```python
from build123d import *

# Parameters (mm, degrees)
F0_W          = 177.334
F0_H          = 19.05
F0_R          = 3.1369
F0_R_2        = 4.7625
F1_DEPTH      = 12.7
F2_W          = 177.334
F2_H          = 6.35
F3_DEPTH      = 25.4
F3_DEPTH_BACK = 12.7


with BuildPart() as f1:
    # F0 (on Front) → F1 (new body)
    with BuildSketch(Plane.XZ):
        with Locations((88.667, 9.525)):
            Rectangle(F0_W, F0_H)
        with Locations((12.467, 9.525)):
            Circle(F0_R, mode=Mode.SUBTRACT)
        with Locations((164.867, 9.525)):
            Circle(F0_R_2, mode=Mode.SUBTRACT)
    extrude(amount=F1_DEPTH)

    # F2 (on face) → F3 (join, two sides)
    with BuildSketch(Plane.XZ.offset(12.7)) as f3_sk:
        with Locations((88.667, 22.225)):
            Rectangle(F2_W, F2_H)
    extrude(amount=F3_DEPTH)
    extrude(f3_sk.sketch, amount=-F3_DEPTH_BACK)


solid = f1.part
```
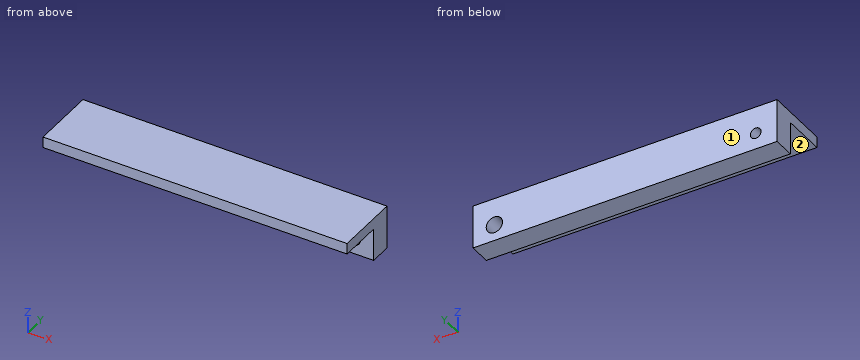
Part model, mm, in its own coordinate system. Face numbers are marked on the shaded views. A direction names the side the tool comes from. Round coordinates to 2 decimals unless told otherwise and drop trailing zeros. Write each loop counter-clockwise with the first axis right and the second up, starting at its lowest first coordinate (ties: lowest second). Pieces come first, ordered by that corner, then holes. Notation, with made-up numbers: M 63,10.5 L 116,10.5 A33 cw 116,40.5 Z; hole C -31,42.5 d7. An arc over 180 degrees is marked long. Answer as CSV lines item,"result". Start each with the question number.
1) Band-saw the part on D-D (z = 16.25). List the corners of the cut face in (x, y).
2) Band-saw the part on B-B (x = 144). List the corners of the cut face in (y, z).
3) Band-saw the part on A-A (y = -10). List the corners of the cut face in (x, z) (1 decimal).
4) Which spindle directions (+Z, -Z, +X, -X, +Y, -Y) get a long thin tool onto all of the face, cutting with end or side? Do the marked faces 1 and 2. Say none if no direction does.
5) Drop flat-ended pins along their axis: pin 1 (6 mm diameter, centred on x = 31, z = 16, fed in from -Y); pin 2 (7.5 mm diameter, centred on x = 60, y = -20, fed in from -Z). Give the stop position or say it passes through.
6) Band-saw the part on C-C (y = -23.5). List the corners of the cut face in (x, z).
7) Drill centre lines: L1, parallel to X at y = -6, z = 7.5; L2, parallel to Y at x = 141.5, z = 17; L3, parallel to Z at x = 14, y = -27.5. Where is each one in solid material? Low to high.
Worked out:
1,outline,"M 0,-12.7 L 177.33,-12.7 L 177.33,0 L 0,0 Z"
2,outline,"M -38.1,19.05 L -12.7,19.05 L -12.7,0 L 0,0 L 0,25.4 L -38.1,25.4 Z"
3,outline,"M 0,0 L 177.3,0 L 177.3,25.4 L 0,25.4 Z; hole C 12.5,9.5 d6.3; hole C 164.9,9.5 d9.5"
4,face 1,"+Z, -Z, +X, -X, +Y"
4,face 2,"-Z, +X, -X, -Y"
5,pin 1,"y = -12.7"
5,pin 2,"z = 19.05"
6,outline,"M 0,19.05 L 177.33,19.05 L 177.33,25.4 L 0,25.4 Z"
7,L1,"0 to 10.07, 14.86 to 160.56, 169.18 to 177.33"
7,L2,"-12.7 to 0"
7,L3,"19.05 to 25.4"
